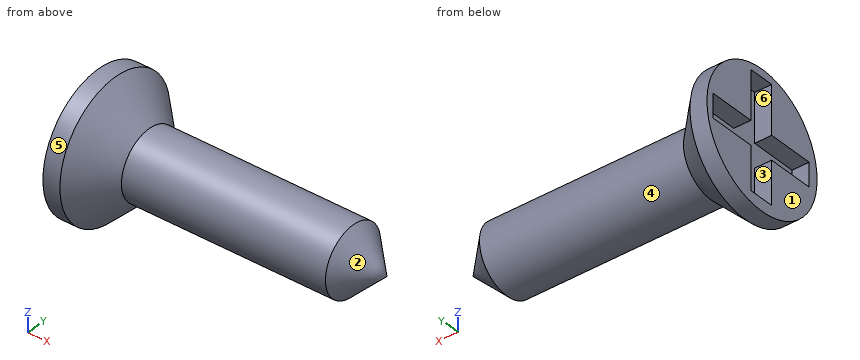
Autodesk Inventor part; units mm, degrees
ref_plane "YZ Plane" through (0, 0, 0) normal (1, 0, 0) x (0, 1, 0)
ref_plane "XZ Plane" through (0, 0, 0) normal (0, 1, 0) x (-1, 0, 0)
ref_plane "XY Plane" through (0, 0, 0) normal (0, 0, 1) x (1, 0, 0)
sketch "Sketch1" plane through (0, 0, 0) normal (1, 0, 0) x (0, 1, 0)
  circle A0 centre (169.2255, 363.3555) radius 48.0965
  circle A1 centre (138.8493, 276.6293) radius 6.35
  point P0 (0, 0)
  dimension "d0" = 12.7
extrude "Extrusion1" add sketch "Sketch1" along normal blind 4.7625 contours A1
chamfer "Chamfer1" distance 3.175 angle 45 1 edges at (4.7625, 132.4993, 276.6293)
sketch "Sketch2" plane through (4.7625, 138.8493, 276.6293) normal (1, 0, 0) x (0, 0, -1)
  circle A0 centre (0, 0) radius 3.175
  circle A1 centre (0, 0) radius 3.175
  point P0 (276.6293, -138.8493)
extrude "Extrusion2" add sketch "Sketch2" along normal blind 22.225
chamfer "Chamfer2" distance 3.175 angle 45 1 edges at (26.9875, 138.8493, 279.8043)
sketch "Sketch3" plane through (0, 138.8493, 276.6293) normal (-1, 0, 0) x (0, 0, 1)
  point P0 (-276.6293, -138.8493)
thread "Thread1"
sketch "Sketch4" plane through (0, 138.8493, 276.6293) normal (-1, 0, 0) x (0, 0, 1)
  line L0 (-1.16, 5.6468) -> (1.058, 5.6468)
  line L1 (1.058, 5.6468) -> (1.058, -5.4225)
  line L2 (1.058, -5.4225) -> (-1.16, -5.4225)
  line L3 (-1.16, -5.4225) -> (-1.16, 5.6468)
  line L4 (-5.2022, 1.2937) -> (5.5977, 1.2937)
  line L5 (5.5977, 1.2937) -> (5.5977, -1.1109)
  line L6 (5.5977, -1.1109) -> (-5.2022, -1.1109)
  line L7 (-5.2022, -1.1109) -> (-5.2022, 1.2937)
  point P0 (-276.6293, -138.8493)
extrude "Extrusion3" cut sketch "Sketch4" against normal blind 1.5875
properties part number "screw"
Geometry check sheet. Reference: the model listing, model coordinates, mm. Face numbers are marked on the shaded views. A direction names the side the tool comes from. Round coordinates to 2 decimals unless told otherwise and drop trailing zeros. Order: outer loops, then holes, each group sorted by start corner. A loop starts at its lowest first (then second) coordinate and runs counter-clockwise, first axis right, second up. Notation, with made-up numbers: (-21.75, -16.75) - (22.25, -16.75) arc R20 cw to (22.25, 9.25) - close; hole circle Ø10 at (56, 9.5). An arc over 180 degrees is marked (long way). Use a Markdown table: item, result. Add a question column.
(1) Depth check by flat-ended pin: pin 1 (5 mm diameter, centred on y = 142.5, z = 279.5, fed in from -X); pin 2 (5 mm diameter, centred on x = 21.5, z = 280, fed in from -Y); pin 3 (0.8 mm diameter, centred on x = 0.5, y = 139.5, fed in from +Z); pin 4 (0.5 mm diameter, centred on x = 0.5, z = 273.5, fed in from -Y). Enter the tip coordinate at first touch or a pass-through.
(2) Release check for a two-part mould opening along Z. For the marked faces 1, 2 and 3 record: pulls with the +Z half, pulls with the -Z half, needs draft (parallel to the pull), parting line crosses it, or undercut.
(3) Sectioned sample at B-B, the plane x = 25. Enter the section's corners in (y, z) (1 decimal), and give its area (3 significant figures).
(4) Material ranges on line 1 along Z through (x, y) = (6.5, 136.25); line 2 along Y through (x, z) = (23.25, 274.25); line 3 along Z through (x, y) = (11.5, 136.75), recorded low to high. Write a range as [from, to].
(5) Tool access check on the marked faces 4, 5 and 6. Record the directions out of +Z, -Z, +X, -X, +Y, -Y that give a thin tool (end or side, any length) a straight path to the whole face; none if there is none.
(6) Sectioned sample at A-A, the plane x = 14.5. Enter the section's corners in (y, z) (3 decimals).
Answers below:
| question | item | result |
|---|---|---|
| 1 | pin 1 | x = 0 |
| 1 | pin 2 | y = 135.8 |
| 1 | pin 3 | z = 282.97 |
| 1 | pin 4 | y = 133.19 |
| 2 | face 1 | needs draft |
| 2 | face 2 | parting line crosses it |
| 2 | face 3 | undercut |
| 3 | outline | circle Ø4 at (138.8, 276.6) |
| 3 | area | 12.4 mm² |
| 4 | line 1 | [274.81, 278.45] |
| 4 | line 2 | [136.75, 140.95] |
| 4 | line 3 | [274.25, 279.01] |
| 5 | face 4 | +X |
| 5 | face 5 | +X, -X |
| 5 | face 6 | -X |
| 6 | outline | circle Ø6.35 at (138.849, 276.629) |
